```python
from build123d import *

# Parameters (mm, degrees)
SKETCH1_R            = 20
BOSS_EXTRUDE1_DEPTH  = 4
BOSS_EXTRUDE2_START  = -2.4
BOSS_EXTRUDE2_DEPTH  = 2.4
SKETCH6_W            = 60
SKETCH6_H            = 10
BOSS_EXTRUDE5_DEPTH  = 5
SKETCH7_R            = 0.75
CUT_EXTRUDE1_DEPTH   = 5
SKETCH8_W            = 5
SKETCH8_H            = 10
BOSS_EXTRUDE6_DEPTH  = 20
SKETCH9_W            = 21.637597824
SKETCH9_H            = 14.8
SKETCH9_R            = 1.6
BOSS_EXTRUDE7_DEPTH  = 5
SKETCH10_W           = 12.4
SKETCH10_H           = 22.64948999
CUT_EXTRUDE2_DEPTH   = 75.256312863
SKETCH11_R           = 0.6
CUT_EXTRUDE3_DEPTH   = 10
SKETCH12_R           = 4.5
CUT_EXTRUDE4_DEPTH   = 5
SKETCH14_W           = 5
SKETCH14_H           = 10
BOSS_EXTRUDE9_DEPTH  = 21
SKETCH15_R           = 1.7
BOSS_EXTRUDE10_DEPTH = 6


with BuildPart() as part:
    # Sketch1 → Boss-Extrude1 (new body)
    with BuildSketch(Plane.XY):
        Circle(SKETCH1_R)
        with BuildLine():
            Line((-14.05, 2), (-2.209072203, 2.65))
            ThreePointArc((-2.209072203, 2.65), (0, 3.45), (2.209072203, 2.65))
            Line((2.209072203, 2.65), (14.05, 2))
            ThreePointArc((14.05, 2), (16.05, 0), (14.05, -2))
            Line((14.05, -2), (2.209072203, -2.65))
            ThreePointArc((2.209072203, -2.65), (0, -3.45), (-2.209072203, -2.65))
            Line((-2.209072203, -2.65), (-14.05, -2))
            ThreePointArc((-14.05, -2), (-16.05, 0), (-14.05, 2))
        make_face(mode=Mode.SUBTRACT)
    extrude(amount=-BOSS_EXTRUDE1_DEPTH)

    # Sketch2 → Boss-Extrude2 (add)
    with BuildSketch(Plane(origin=(0, 0, -4), x_dir=(-1, 0, 0), z_dir=(0, 0, -1)).offset(BOSS_EXTRUDE2_START)):
        with BuildLine():
            Line((14.05, 2), (2.209072203, 2.65))
            ThreePointArc((2.209072203, 2.65), (3.45, 0), (2.209072203, -2.65))
            Line((2.209072203, -2.65), (14.05, -2))
            ThreePointArc((14.05, -2), (16.05, 0), (14.05, 2))
        make_face()
        with BuildLine():
            Line((-2.209072203, -2.65), (-14.05, -2))
            ThreePointArc((-14.05, -2), (-16.05, 0), (-14.05, 2))
            Line((-14.05, 2), (-2.209072203, 2.65))
            ThreePointArc((-2.209072203, 2.65), (-3.45, 0), (-2.209072203, -2.65))
        make_face()
    extrude(amount=BOSS_EXTRUDE2_DEPTH)

    # Sketch6 → Boss-Extrude5 (add)
    with BuildSketch(Plane.XY):
        with Locations((-37, 13)):
            Rectangle(SKETCH6_W, SKETCH6_H)
        with Locations((-37, -13)):
            Rectangle(SKETCH6_W, SKETCH6_H)
    extrude(amount=BOSS_EXTRUDE5_DEPTH)

    # Sketch7 → Cut-Extrude1 (cut)
    with BuildSketch(Plane(origin=(0, 0, 0), x_dir=(-1, 0, 0), z_dir=(0, 0, -1))):
        with Locations((56.078339908, 15.85)):
            Circle(SKETCH7_R)
        with Locations((56.078339908, -11.95)):
            Circle(SKETCH7_R)
    extrude(amount=-CUT_EXTRUDE1_DEPTH, mode=Mode.SUBTRACT)

    # Sketch8 → Boss-Extrude6 (add)
    with BuildSketch(Plane.XY.offset(5)):
        with Locations((-41.629269641, 13)):
            Rectangle(SKETCH8_W, SKETCH8_H)
    extrude(amount=BOSS_EXTRUDE6_DEPTH)

    # Sketch9 → Boss-Extrude7 (add)
    with BuildSketch(Plane.XY.offset(25)):
        with Locations((-49.948068553, 10.6)):
            Rectangle(SKETCH9_W, SKETCH9_H)
        with Locations((-55.565935261, 7.090653296)):
            Circle(SKETCH9_R, mode=Mode.SUBTRACT)
    extrude(amount=BOSS_EXTRUDE7_DEPTH)

    # Sketch10 → Cut-Extrude2 (cut, through all)
    with BuildSketch(Plane.XY.offset(5)):
        with Locations((-56.078339908, 1.875255005)):
            Rectangle(SKETCH10_W, SKETCH10_H)
    extrude(amount=-CUT_EXTRUDE2_DEPTH, mode=Mode.SUBTRACT)

    # Sketch11 → Cut-Extrude3 (cut)
    with BuildSketch(Plane.XY):
        with Locations((-10.45, 0)):
            Circle(SKETCH11_R)
        with Locations((10.45, 0)):
            Circle(SKETCH11_R)
    extrude(amount=-CUT_EXTRUDE3_DEPTH, mode=Mode.SUBTRACT)

    # Sketch12 → Cut-Extrude4 (cut)
    with BuildSketch(Plane(origin=(0, 0, -4), x_dir=(-1, 0, 0), z_dir=(0, 0, -1))):
        Circle(SKETCH12_R)
    extrude(amount=-CUT_EXTRUDE4_DEPTH, mode=Mode.SUBTRACT)

    # Sketch14 → Boss-Extrude9 (add)
    with BuildSketch(Plane.XY.offset(5)):
        with Locations((-26.615087819, -13)):
            Rectangle(SKETCH14_W, SKETCH14_H)
    extrude(amount=BOSS_EXTRUDE9_DEPTH)

    # Sketch15 → Boss-Extrude10 (add)
    with BuildSketch(Plane.XY.offset(26)):
        with BuildLine():
            Line((-29.115087819, -8), (-2.104852737, 4.535371535))
            ThreePointArc((-2.104852737, 4.535371535), (4.663893683, 1.802247406), (1.491850027, -4.772251408))
            Line((1.491850027, -4.772251408), (-24.115087819, -18))
            Line((-24.115087819, -18), (-29.115087819, -18))
            Line((-29.115087819, -18), (-29.115087819, -8))
        make_face()
        Circle(SKETCH15_R, mode=Mode.SUBTRACT)
    extrude(amount=-BOSS_EXTRUDE10_DEPTH)


solid = part.part
```
Design review of the part built by this model. Coordinates are the model's own, in mm. A direction names the side the tool comes from. Coordinates: 2 decimals unless noted, no trailing zeros. Order: outer loops, then holes, each group sorted by start corner. A loop starts at its lowest first (then second) coordinate and runs counter-clockwise, first axis right, second up. Notation, with made-up numbers: M 58,-4.5 L 105,-4.5 A8 cw 105,4.5 Z; hole C 82.5,45.25 d7. An arc over 180 degrees is marked long. Answer as a JSON object with one key per item and string values. Group by question number.
1) Tool access review of faces 5 (the flat face through (-16, -13, 5)), 6 (the flat face through (-65, -8, 2)), 7 (the flat face through (-56, 14, 5)), 8 (the flat face through (-48, -13, 5)): name each direction out of +Z, -Z, +X, -X, +Y, -Y from which nothing blocks a thin tool from reaching the whole face with its end or side.
2) Add section C-C, the plane x = 0. Write out the cut boundary in (y, z), then the cut area to 3 significant figures.
3) Add section B-B, the plane z = 8.5. Write out the cut boundary in (x, y), then the cut area to 3 significant figures.
4) Mouldability with a two-part tool opening along X and no side actions: class faces 1 (the cylindrical face through (16.05, 0.04, -0.79)), 2 (the flat face through (-50, 11, 30)), 3 (the flat face through (-29.115, -13, 15)), 4 (the flat face through (-62.278, 11, 3)) as pulls with the +X half, pulls with the -X half, needs draft (parallel to the pull), parting line crosses it, or undercut.
5) Add section A-A, the plane x = -33. Write out the cut boundary in (y, z), then the cut area to 3 significant figures.
6) Wall thickness on L1, parallel to Z at x = -14.5, y = -5; L2, parallel to Y at x = -9, z = 1; L3, parallel to Z at x = -19.5, y = -13: over which ranges is each line inside the solid? List them lowest first.
7) Add section D-D, the plane x = -43. Write out the cut boundary in (y, z).
8) For pin 1 (3 mm diameter, centred on x = -23.5, z = 23.5, fed in from -Y); pin 2 (11.5 mm diameter, centred on x = 0, y = 0, fed in from +Z); pin 3 (3 mm diameter, centred on y = -13.5, z = 13.5, fed in from -X), all flat-tipped, find the tip position at first contact; note any pin that passes through.
Computed values:
{
 "1": {"face 5": "+X, +Y, -Y", "face 6": "+Z, -Z, +X, -X", "face 7": "-X, +Y, -Y", "face 8": "+Z, -X, -Y"},
 "2": {"outline": "M -20,-4 L -4.5,-4 L -4.5,0 L -20,0 Z; M -5.54,20 L -1.7,20 L -1.7,26 L -5.54,26 Z; M 1.7,20 L 5,20 L 5,26 L 1.7,26 Z; M 4.5,-4 L 20,-4 L 20,0 L 4.5,0 Z", "area": "167 mm^2"},
 "3": {"outline": "M -44.13,8 L -39.13,8 L -39.13,18 L -44.13,18 Z; M -29.12,-18 L -24.12,-18 L -24.12,-8 L -29.12,-8 Z", "area": "100 mm^2"},
 "4": {"face 1": "undercut", "face 2": "needs draft", "face 3": "pulls with the -X half", "face 4": "undercut"},
 "5": {"outline": "M -18,0 L -8,0 L -8,5 L -18,5 Z; M 8,0 L 18,0 L 18,5 L 8,5 Z", "area": "100 mm^2"},
 "6": {"L1": "z = -4 to 0, 20 to 26", "L2": "y = -18 to -8, 8 to 18", "L3": "z = 0 to 5, 20 to 26"},
 "7": {"outline": "M -18,0 L -8,0 L -8,5 L -18,5 Z; M 3.2,25 L 8,25 L 8,0 L 18,0 L 18,30 L 3.2,30 Z"},
 "8": {"pin 1": "stops at y = -18", "pin 2": "stops at z = 26", "pin 3": "stops at x = -29.12"}
}
